Part model, mm, in its own coordinate system. Face numbers are marked on the shaded views. A direction names the side the tool comes from. Coordinates: 2 decimals unless noted, no trailing zeros. Write each loop counter-clockwise with the first axis right and the second up, starting at its lowest first coordinate (ties: lowest second). Pieces come first, ordered by that corner, then holes. Notation, with made-up numbers: (-30, 79.25) -> (6, 79.25) arc R22 ccw to (6, 89.25) -> close; hole circle Ø11 at (25, 28). An arc over 180 degrees is marked (long way). Write item = value, one per line.
from build123d import *

# Parameters (mm, degrees)
F0_W     = 31.75
F0_H     = 31.75
F1_DEPTH = 19.05
F2_W     = 19.05
F2_H     = 19.05
F3_DEPTH = 19.051
F5_D     = 5.6134
F5_DEPTH = 7.62


with BuildPart() as f1:
    # F0 (on Front) → F1 (new body)
    with BuildSketch(Plane.XZ):
        with Locations((15.875, -15.875)):
            Rectangle(F0_W, F0_H)
    extrude(amount=F1_DEPTH)

    # F2 (on face) → F3 (cut, through all)
    with BuildSketch(Plane.XZ.offset(19.05)):
        with Locations((15.875, -9.525)):
            Rectangle(F2_W, F2_H)
    extrude(amount=-F3_DEPTH, mode=Mode.SUBTRACT)

    # F5
    with Locations(Plane.YZ.offset(31.75)):
        with Locations((-9.525, -9.652)):
            Hole(F5_D / 2, depth=F5_DEPTH)


solid = f1.part
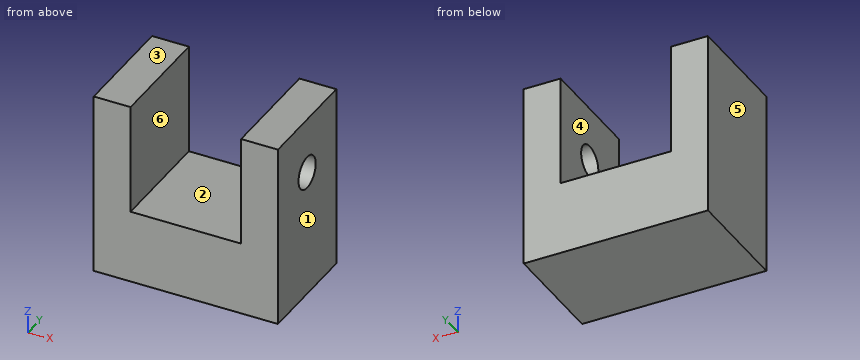
Q1. Which spindle directions (+Z, -Z, +X, -X, +Y, -Y) get a long thin tool onto all of the face, cutting with end or side? Do the marked faces 1 and 2. Say none if no direction does.
Model answer:
face_1 = +Z, -Z, +X, +Y, -Y
face_2 = +Z, +Y, -Y
Q2. Probe line 1 (X direction, y = -12.5, z = -13); line 2 (Z direction, x = 10, y = -9.75); line 3 (X direction, y = -11, z = -12). List the from-to ranges inside material, lowest first. Write a range as from..to.
Model answer:
line_1 = 0..6.35, 25.4..31.75
line_2 = -31.75..-19.05
line_3 = 0..6.35
Q3. Pin check, flat tips, straight feed: pin 1 (8 mm diameter, centred on x = 13.5, z = -9, fed in from -Y); pin 2 (9.5 mm diameter, centred on x = 19.5, y = -5.5, fed in from +Z); pin 3 (3.5 mm diameter, centred on y = -9.525, z = -9.652, fed in from +X). Stop position of each tip, or through.
Model answer:
pin_1 = through
pin_2 = -19.05
pin_3 = 6.35
Q4. Mould opens along X. For the marked faces 3, 4, 5 and 6 say: released by +X, released by -X, zero draft, split by the parting line, or undercut.
Model answer:
face_3 = zero draft
face_4 = undercut
face_5 = released by -X
face_6 = undercut
Q5. Saw through at C-C on x = 27. Give the cut face in (y, z) (3 decimals), and give its area (3 significant figures).
Model answer:
outline = (-19.05, -31.75) -> (0, -31.75) -> (0, 0) -> (-19.05, 0) -> close; hole circle Ø5.613 at (-9.525, -9.652)
area = 580 mm²
Q6. Saw through at B-B on y = -11. Give the cut face in (x, z), and give its area (3 significant figures).
Model answer:
outline = (0, -31.75) -> (31.75, -31.75) -> (31.75, -12.04) -> (25.4, -12.04) -> (25.4, -19.05) -> (6.35, -19.05) -> (6.35, 0) -> (0, 0) -> close; (25.4, -7.26) -> (31.75, -7.26) -> (31.75, 0) -> (25.4, 0) -> close
area = 615 mm²
Q7. Saw through at D-D on y = -16. Give the cut face in (x, z).
Model answer:
outline = (0, -31.75) -> (31.75, -31.75) -> (31.75, 0) -> (25.4, 0) -> (25.4, -19.05) -> (6.35, -19.05) -> (6.35, 0) -> (0, 0) -> close
Q8. Saw through at A-A on z = -13. Give the cut face in (x, y).
Model answer:
outline = (0, -19.05) -> (6.35, -19.05) -> (6.35, 0) -> (0, 0) -> close; (25.4, -19.05) -> (31.75, -19.05) -> (31.75, 0) -> (25.4, 0) -> close
